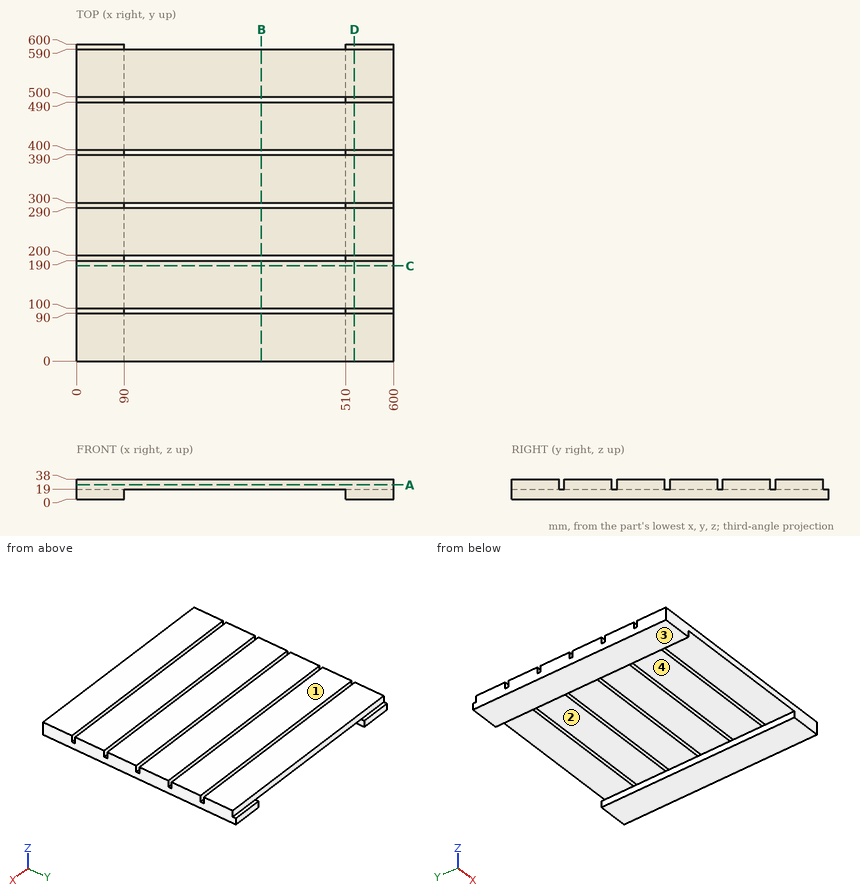
Here's the drawing with two shaded views (mm, measured from the low corner). I have some questions. A direction names the side the tool comes from. Round coordinates to 2 decimals unless told otherwise and drop trailing zeros. Order: outer loops, then holes, each group sorted by start corner. A loop starts at its lowest first (then second) coordinate and runs counter-clockwise, first axis right, second up. Notation, with made-up numbers: (-25, 3.5) -> (10, 3.5) arc R27 cw to (10, 37.5) -> close; hole circle Ø2 at (-34.5, 43.5). An arc over 180 degrees is marked (long way). Use a Markdown table: item, result. Add a question column.
(1) Suppose I cut it at B-B, the plane x = 350. Please give me the cut outline in (y, z).
(2) For the marked faces 1 and 2, which set-ups out of +Z, -Z, +X, -X, +Y, -Y let a thin tool reach every point of the face, with its end or its side?
(3) For pin 1 Ø15 at (x, z) = (280.5, 30.5) entering from +Y; pin 2 Ø3 at (x, y) = (533, 396) entering from +Z; pin 3 Ø2 at (x, y) = (88, 173) entering from -Z; pin 4 Ø1.5 at (x, y) = (473.5, 407.5) entering from -Z, each with a flat end and sliding along its axis, tell me the tip position at first contact or that it passes through.
(4) If we mould it in two halves opening along X, with no side actions, what happens to the marked faces 3 and 4? For each: released by +X, released by -X, zero draft, split by the parting line, or undercut.
(5) Suppose I cut it at D-D, the plane x = 526. Please give me the cut outline in (y, z), and give its area (3 significant figures).
(6) I need wall thicknesses on line 1 along Y through (x, z) = (209.5, 32.5); line 2 along X through (y, z) = (502, 5.5); line 3 along Z through (x, y) = (311, 142.5). Which ranges of each line are inside material? Lowest first, please.
(7) Suppose I cut it at C-C, the plane y = 180. Please give me the cut outline in (x, z), and give its area (3 significant figures).
(8) Suppose I cut it at A-A, the plane z = 27. Please give me the cut outline in (x, y), and give its area (3 significant figures).
Verdict:
| question | item | result |
|---|---|---|
| 1 | outline | (0, 19) -> (90, 19) -> (90, 38) -> (0, 38) -> close; (100, 19) -> (190, 19) -> (190, 38) -> (100, 38) -> close; (200, 19) -> (290, 19) -> (290, 38) -> (200, 38) -> close; (300, 19) -> (390, 19) -> (390, 38) -> (300, 38) -> close; (400, 19) -> (490, 19) -> (490, 38) -> (400, 38) -> close; (500, 19) -> (590, 19) -> (590, 38) -> (500, 38) -> close |
| 2 | face 1 | +Z, +X, -X, +Y, -Y |
| 2 | face 2 | -Z, +Y, -Y |
| 3 | pin 1 | y = 590 |
| 3 | pin 2 | z = 19 |
| 3 | pin 3 | z = 0 |
| 3 | pin 4 | z = 19 |
| 4 | face 3 | zero draft |
| 4 | face 4 | undercut |
| 5 | outline | (0, 0) -> (600, 0) -> (600, 19) -> (590, 19) -> (590, 38) -> (500, 38) -> (500, 19) -> (490, 19) -> (490, 38) -> (400, 38) -> (400, 19) -> (390, 19) -> (390, 38) -> (300, 38) -> (300, 19) -> (290, 19) -> (290, 38) -> (200, 38) -> (200, 19) -> (190, 19) -> (190, 38) -> (100, 38) -> (100, 19) -> (90, 19) -> (90, 38) -> (0, 38) -> close |
| 5 | area | 21,700 mm2 |
| 6 | line 1 | 0 to 90, 100 to 190, 200 to 290, 300 to 390, 400 to 490, 500 to 590 |
| 6 | line 2 | 0 to 90, 510 to 600 |
| 6 | line 3 | 19 to 38 |
| 7 | outline | (0, 0) -> (90, 0) -> (90, 19) -> (510, 19) -> (510, 0) -> (600, 0) -> (600, 38) -> (0, 38) -> close |
| 7 | area | 14,800 mm2 |
| 8 | outline | (0, 0) -> (600, 0) -> (600, 90) -> (0, 90) -> close; (0, 100) -> (600, 100) -> (600, 190) -> (0, 190) -> close; (0, 200) -> (600, 200) -> (600, 290) -> (0, 290) -> close; (0, 300) -> (600, 300) -> (600, 390) -> (0, 390) -> close; (0, 400) -> (600, 400) -> (600, 490) -> (0, 490) -> close; (0, 500) -> (600, 500) -> (600, 590) -> (0, 590) -> close |
| 8 | area | 324,000 mm2 |
